Geometry check sheet. Reference: the model listing, model coordinates, mm. Coordinates: 2 decimals unless noted, no trailing zeros. Loops run counter-clockwise (first coordinate to the right, second up) from the corner with the lowest first, then second, coordinate; pieces in that order, holes last.
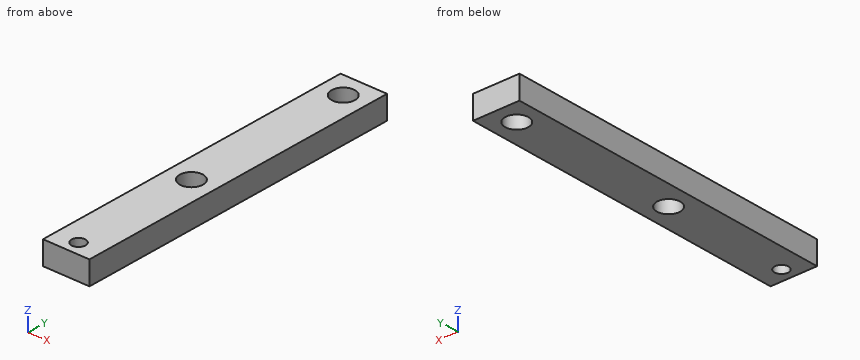
from build123d import *

# Parameters (mm, degrees)
SKETCH1_W           = 10
SKETCH1_H           = 72.5
BOSS_EXTRUDE1_DEPTH = 5
SKETCH2_R           = 2.5
CUT_EXTRUDE1_DEPTH  = 6
SKETCH3_R           = 1.5
SKETCH3_R_2         = 2.5
CUT_EXTRUDE2_DEPTH  = 6


with BuildPart() as part:
    # Sketch1 → Boss-Extrude1 (new body)
    with BuildSketch(Plane.XY):
        with Locations((-5, 36.25)):
            Rectangle(SKETCH1_W, SKETCH1_H)
    extrude(amount=BOSS_EXTRUDE1_DEPTH)

    # Sketch2 → Cut-Extrude1 (cut, through all)
    with BuildSketch(Plane.XY.offset(5)):
        with Locations((-5, 67.5)):
            Circle(SKETCH2_R)
    extrude(amount=-CUT_EXTRUDE1_DEPTH, mode=Mode.SUBTRACT)

    # Sketch3 → Cut-Extrude2 (cut, through all)
    with BuildSketch(Plane.XY.offset(5)):
        with Locations((-5, 3)):
            Circle(SKETCH3_R)
        with Locations((-5, 30.5)):
            Circle(SKETCH3_R_2)
    extrude(amount=-CUT_EXTRUDE2_DEPTH, mode=Mode.SUBTRACT)


solid = part.part
1) Material ranges on probe 1 along Y at (x, z) = (-5, 3.85); probe 2 along Y at (x, z) = (-4, 0.4); probe 3 along Y at (x, z) = (-3, 2.85), recorded low to high.
Data:
probe 1: y = 0 to 1.5, 4.5 to 28, 33 to 65, 70 to 72.5
probe 2: y = 0 to 1.88, 4.12 to 28.21, 32.79 to 65.21, 69.79 to 72.5
probe 3: y = 0 to 29, 32 to 66, 69 to 72.5
2) Section check D-D on y = 30.5. Record the cut outline in (x, z), and give its area (3 significant figures).
Data:
outline: (-10, 0) - (-7.5, 0) - (-7.5, 5) - (-10, 5) - close; (-2.5, 0) - (0, 0) - (0, 5) - (-2.5, 5) - close
area: 25.0 mm2
3) Section check B-B on z = 2.3. Record the cut outline in (x, y), and give its area (3 significant figures).
Data:
outline: (-10, 0) - (0, 0) - (0, 72.5) - (-10, 72.5) - close; hole circle Ø5 at (-5, 30.5); hole circle Ø5 at (-5, 67.5); hole circle Ø3 at (-5, 3)
area: 679 mm2
4) Section check A-A on x = -5. Record the cut outline in (y, z), and give its area (4 significant figures).
Data:
outline: (0, 0) - (1.5, 0) - (1.5, 5) - (0, 5) - close; (4.5, 0) - (28, 0) - (28, 5) - (4.5, 5) - close; (33, 0) - (65, 0) - (65, 5) - (33, 5) - close; (70, 0) - (72.5, 0) - (72.5, 5) - (70, 5) - close
area: 297.5 mm2
5) Section check C-C on y = 3. Record the cut outline in (x, z), and give its area (3 significant figures).
Data:
outline: (-10, 0) - (-6.5, 0) - (-6.5, 5) - (-10, 5) - close; (-3.5, 0) - (0, 0) - (0, 5) - (-3.5, 5) - close
area: 35.0 mm2
